Read the model definition and answer for the solid it produces. Units are mm, in the model's axes. Face numbers are marked on the shaded views. A direction names the side the tool comes from. Coordinates: 2 decimals unless noted, no trailing zeros. Loops run counter-clockwise (first coordinate to the right, second up) from the corner with the lowest first, then second, coordinate; pieces in that order, holes last. Notation, with made-up numbers: (58.5, 23.5) -> (100.5, 23.5) arc R16 cw to (100.5, 42.5) -> close; hole circle Ø4 at (86.25, 20). An arc over 180 degrees is marked (long way). Answer as a JSON object with one key per item and string values. Group by question number.
1) Section B-B, the plane x = 39 is taken. Give the vertices of the cut face in (y, z).
2) Consider probe 1 along X at (y, z) = (49.5, 0); probe 2 along Z at (x, y) = (0, 24.2); probe 3 along Z at (x, y) = (39, 31). Determine where each line is inside the solid, lowest interval first. Write a range as [from, to].
3) Determine the mould class of the marked faces 6, 7 and 8 for opening direction Z: released by +Z, released by -Z, zero draft, split by the parting line, or undercut.
4) Flat-ended cylindrical pins translate along their axes: P1, Ø2, axis at y = 34.5, z = -2, coming from the +X side; P2, Ø7, axis at x = 0, z = 0, coming from the +Y side; P3, Ø8, axis at y = 8.5, z = -8, coming from the -X side. Find the tip coordinate at first contact, or state that the pin passes through.
5) Section A-A, the plane y = 55.5 is taken. Give the vertices of the cut face in (x, z), plus the area to 3 significant figures.
6) Which of the six approach directions +Z, -Z, +X, -X, +Y, -Y give full straight-line access (tool end or side, diameter ignored) to the marked faces 1, 2, 3, 4 and 5?
7) Section D-D, the plane y = 6.5 is taken. Give the vertices of the cut face in (x, z), plus the area to 3 significant figures.
8) Section C-C, the plane x = 66 is taken. Give the vertices of the cut face in (y, z).
from build123d import *

# Parameters (mm, degrees)
BOSS_EXTRUDE1_DEPTH = 23
BOSS_EXTRUDE2_START = -14
BOSS_EXTRUDE2_DEPTH = 68
CUT_EXTRUDE1_DEPTH  = 34
SKETCH4_R           = 6
CUT_EXTRUDE2_DEPTH  = 127.368508735
SKETCH5_W           = 28
SKETCH5_H           = 28
CUT_EXTRUDE3_DEPTH  = 10
CUT_EXTRUDE4_DEPTH  = 16
CUT_EXTRUDE5_DEPTH  = 120.419428905
FILLET1_R           = 8


with BuildPart() as part:
    # Sketch1 → Boss-Extrude1 (new, symmetric)
    with BuildSketch(Plane.XY):
        Polygon((104, 0), (-104, 0), (-99.985564599, 14), (99.985564599, 14), align=None)
    extrude(amount=BOSS_EXTRUDE1_DEPTH, both=True)

    # Sketch2 → Boss-Extrude2 (add)
    with BuildSketch(Plane(origin=(0, 14, 0), x_dir=(1, 0, 0), z_dir=(0, 1, 0)).offset(BOSS_EXTRUDE2_START)):
        with BuildLine():
            Line((48.856934001, 23), (-48.856934001, 23))
            ThreePointArc((-48.856934001, 23), (-54, 0), (-48.856934001, -23))
            Line((-48.856934001, -23), (48.856934001, -23))
            ThreePointArc((48.856934001, -23), (54, 0), (48.856934001, 23))
        make_face()
    extrude(amount=BOSS_EXTRUDE2_DEPTH)

    # Sketch3 → Cut-Extrude1 (cut, symmetric)
    with BuildSketch(Plane.XY):
        with BuildLine():
            Line((-28, 68), (-28, 52))
            Line((-28, 52), (-23.661097096, 52))
            Line((-23.661097096, 52), (-23.661097096, 48))
            ThreePointArc((-23.661097096, 48), (0, 28.019015328), (23.661097096, 48))
            Line((23.661097096, 48), (23.661097096, 52))
            Line((23.661097096, 52), (28, 52))
            Line((28, 52), (28, 68))
            Line((28, 68), (-28, 68))
        make_face()
    extrude(amount=CUT_EXTRUDE1_DEPTH, both=True, mode=Mode.SUBTRACT)

    # Sketch4 → Cut-Extrude2 (cut, through all)
    with BuildSketch(Plane(origin=(0, 68, 0), x_dir=(1, 0, 0), z_dir=(0, 1, 0))):
        with Locations(Location((-39, 0, 0), (0, 0, 270))):
            Circle(SKETCH4_R)
        with Locations(Location((39, 0, 0), (0, 0, 90))):
            Circle(SKETCH4_R)
    extrude(amount=-CUT_EXTRUDE2_DEPTH, mode=Mode.SUBTRACT)

    # Sketch5 → Cut-Extrude3 (cut)
    with BuildSketch(Plane.XZ):
        with Locations((-39, 0)):
            Rectangle(SKETCH5_W, SKETCH5_H)
        with Locations((39, 0)):
            Rectangle(SKETCH5_W, SKETCH5_H)
    extrude(amount=-CUT_EXTRUDE3_DEPTH, mode=Mode.SUBTRACT)

    # Sketch6 → Cut-Extrude4 (cut, symmetric)
    with BuildSketch(Plane.XY):
        Polygon((-97.5, 0), (-96.926509228, 2), (96.926509228, 2), (97.5, 0), align=None)
    extrude(amount=CUT_EXTRUDE4_DEPTH, both=True, mode=Mode.SUBTRACT)

    # Sketch7 → Cut-Extrude5 (cut, through all)
    with BuildSketch(Plane(origin=(0, 14, 0), x_dir=(1, 0, 0), z_dir=(0, 1, 0))):
        with BuildLine():
            Line((-85, 6), (-77, 6))
            ThreePointArc((-77, 6), (-71, 0), (-77, -6))
            Line((-77, -6), (-85, -6))
            ThreePointArc((-85, -6), (-91, 0), (-85, 6))
        make_face()
        with BuildLine():
            Line((85, 6), (77, 6))
            ThreePointArc((77, 6), (71, 0), (77, -6))
            Line((77, -6), (85, -6))
            ThreePointArc((85, -6), (91, 0), (85, 6))
        make_face()
    extrude(amount=-CUT_EXTRUDE5_DEPTH, mode=Mode.SUBTRACT)

    # Sketch8 → Cut-Revolve1 (revolve, cut)
    with BuildSketch(Plane.XY, mode=Mode.PRIVATE) as cut_revolve1_sk:
        Polygon((4, 22.422457805), (0, 20.019015328), (0, 28.019015328), (0, 30.422457805), (4, 30.422457805), align=None)
    revolve(cut_revolve1_sk.sketch.rotate(Axis((0, 28.019015328, 0), (0, -1, 0)), 180), axis=Axis((0, 28.019015328, 0), (0, -1, 0)), mode=Mode.SUBTRACT)

    # Fillet1
    fillet1_edges = [part.edges().sort_by_distance(p)[0] for p in [
        (54, 14, 0),
        (-54, 14, 0),
    ]]
    fillet(fillet1_edges, radius=FILLET1_R)


solid = part.part
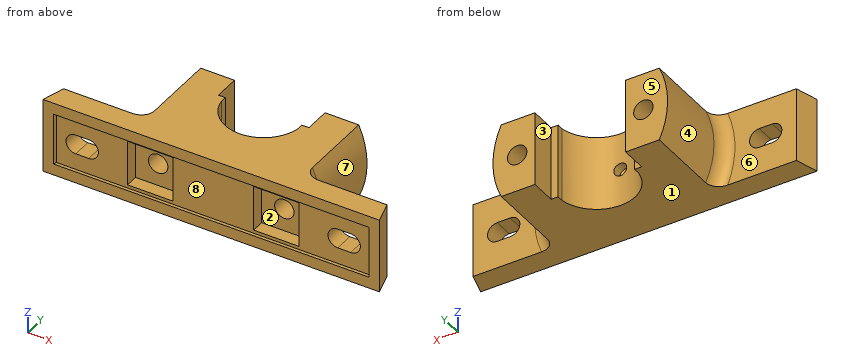
Determined:
{
 "1": {"outline": "(0, -23) -> (68, -23) -> (68, -6) -> (10, -6) -> (10, -14) -> (2, -14) -> (2, -16) -> (0, -16) -> close; (0, 16) -> (2, 16) -> (2, 14) -> (10, 14) -> (10, 6) -> (68, 6) -> (68, 23) -> (0, 23) -> close"},
 "2": {"probe 1": "[-54, -45], [-33, -23.66], [23.66, 33], [45, 54]", "probe 2": "[-23, -4], [4, 23]", "probe 3": "[-23, -6], [6, 23]"},
 "3": {"face 6": "zero draft", "face 7": "split by the parting line", "face 8": "undercut"},
 "4": {"P1": "x = 53.99", "P2": "y = 22.12", "P3": "x = -102.71"},
 "5": {"outline": "(-48.86, -23) -> (-28, -23) -> (-28, 23) -> (-48.86, 23) arc R54 ccw to start; (28, -23) -> (48.86, -23) arc R54 ccw to (48.86, 23) -> (28, 23) -> close; hole circle Ø12 at (-39, 0); hole circle Ø12 at (39, 0)", "area": "2,010 mm²"},
 "6": {"face 1": "-Z, +X, -X, +Y, -Y", "face 2": "-Y", "face 3": "+Z, -Z, +Y", "face 4": "-X, +Y", "face 5": "+Z, -Z, +X, -X, +Y"},
 "7": {"outline": "(-102.14, -23) -> (102.14, -23) -> (102.14, 23) -> (-102.14, 23) -> close; hole (-85, -6) -> (-77, -6) arc R6 ccw to (-77, 6) -> (-85, 6) arc R6 ccw to start; hole (-53, -14) -> (-25, -14) -> (-25, 14) -> (-53, 14) -> close; hole (25, -14) -> (53, -14) -> (53, 14) -> (25, 14) -> close; hole (77, -6) -> (85, -6) arc R6 ccw to (85, 6) -> (77, 6) arc R6 ccw to start", "area": "7,410 mm²"},
 "8": {"outline": "(0, -23) -> (14, -23) -> (14, 23) -> (0, 23) -> (0, 16) -> (2, 16) -> (2, -16) -> (0, -16) -> close"}
}
